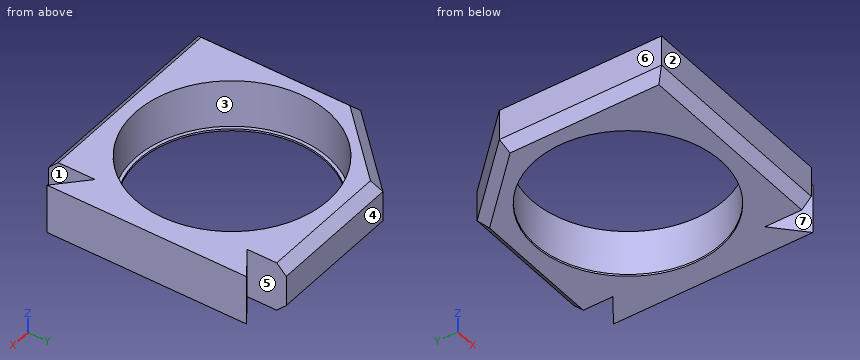
```python
from build123d import *

# Parameters (mm, degrees)
F0_R     = 10.1
F1_DEPTH = 5
F0_R_2   = 9.75
F2_DEPTH = 0.2
F3_SIZE  = 1


with BuildPart() as f1:
    # F0 (on Top) → F1 (new body)
    with BuildSketch(Plane.XY):
        Polygon((-16.0227272727, -12.5188677256), (5.6772727273, -12.5188677256), (5.6772727273, -7.6613227439), (8.6772727273, -10.5188677256), (8.6772727273, 10.3811322744), (5.6772727273, 8.2811322744), (5.6772727273, 12.3811322744), (-8.3227272727, 12.3811322744), (-16.0227272727, 4.4811322744), align=None)
        with Locations((-3.6727272727, -0.0688677256)):
            Circle(F0_R, mode=Mode.SUBTRACT)
    extrude(amount=F1_DEPTH)

    # F0 (on Top) → F2 (join)
    with BuildSketch(Plane.XY):
        Polygon((-16.0227272727, -12.5188677256), (5.6772727273, -12.5188677256), (5.6772727273, -7.6613227439), (8.6772727273, -10.5188677256), (8.6772727273, 10.3811322744), (5.6772727273, 8.2811322744), (5.6772727273, 12.3811322744), (-8.3227272727, 12.3811322744), (-16.0227272727, 4.4811322744), align=None)
        with Locations((-3.6727272727, -0.0688677256)):
            Circle(F0_R, mode=Mode.SUBTRACT)
        with Locations((-3.6727272727, -0.0688677256)):
            Circle(F0_R)
        with Locations((-3.6727272727, -0.0688677256)):
            Circle(F0_R_2, mode=Mode.SUBTRACT)
    extrude(amount=-F2_DEPTH)

    # F3
    f3_edges = [f1.edges().sort_by_distance(p)[0] for p in [
        (-5.172727, -12.518868, 5),
        (-16.022727, -4.018868, 5),
        (-12.172727, 8.431132, 5),
        (-1.322727, 12.381132, 5),
        (-1.322727, 12.381132, -0.2),
        (-12.172727, 8.431132, -0.2),
        (-16.022727, -4.018868, -0.2),
        (-5.172727, -12.518868, -0.2),
    ]]
    chamfer(f3_edges, length=F3_SIZE)


solid = f1.part
```
Check sheet for the modelled part. Datum: model origin and axes. Units: mm. Face numbers are marked on the shaded views. A direction names the side the tool comes from. Give positions to 0.01 mm unless a question says otherwise; leave off trailing zeros. Loops run counter-clockwise (first coordinate to the right, second up) from the corner with the lowest first, then second, coordinate; pieces in that order, holes last. Notation, with made-up numbers: M 86.5,48 L 115.5,48 A21 ccw 115.5,66 Z; hole C 33,6.25 d11. An arc over 180 degrees is marked long. Answer in a Markdown table with one row per item.
1) Cross-section at D-D (y = 5.5). Enter the section's corners in (x, z), plus the area to 3 significant figures.
Solutions:
| item | result |
|---|---|
| outline | M -15.03,0.8 L -13.63,-0.2 L -11.68,-0.2 L -11.68,0 L -12.1,0 L -12.1,5 L -13.63,5 L -15.03,4 Z; M 4.33,-0.2 L 8.68,-0.2 L 8.68,5 L 4.75,5 L 4.75,0 L 4.33,0 Z |
| area | 34.4 mm^2 |
2) Cross-section at C-C (z = 2.9). Enter the section's corners in (x, y), plus the area to 3 significant figures.
Solutions:
| item | result |
|---|---|
| outline | M -16.02,-12.52 L 5.68,-12.52 L 5.68,-7.66 L 8.68,-10.52 L 8.68,10.38 L 5.68,8.28 L 5.68,12.38 L -8.32,12.38 L -16.02,4.48 Z; hole C -3.67,-0.07 d20.2 |
| area | 245 mm^2 |
3) Tool access check on the marked faces 1, 2 and 3. Record the directions out of +Z, -Z, +X, -X, +Y, -Y that give a thin tool (end or side, any length) a straight path to the whole face; none if there is none.
Solutions:
| item | result |
|---|---|
| face 1 | +Z, -Z, -Y |
| face 2 | +Z, -Z, +X, -X, -Y |
| face 3 | +Z |
4) Cross-section at A-A (y = -4.25). Enter the section's corners in (x, z), plus the area to 3 significant figures.
Solutions:
| item | result |
|---|---|
| outline | M -16.02,0.8 L -15.02,-0.2 L -12.48,-0.2 L -12.48,0 L -12.87,0 L -12.87,5 L -15.02,5 L -16.02,4 Z; M 5.14,-0.2 L 8.68,-0.2 L 8.68,5 L 5.52,5 L 5.52,0 L 5.14,0 Z |
| area | 32.0 mm^2 |
5) Mould release check, pull along X, two halves, no side actions. Record for the marked faces 4, 5, 6 and 7: released by +X, released by -X, zero draft, split by the parting line, or undercut.
Solutions:
| item | result |
|---|---|
| face 4 | zero draft |
| face 5 | undercut |
| face 6 | released by -X |
| face 7 | undercut |
6) Cross-section at B-B (x = -3). Enter the section's corners in (y, z).
Solutions:
| item | result |
|---|---|
| outline | M -12.52,0.8 L -11.52,-0.2 L -9.8,-0.2 L -9.8,0 L -10.15,0 L -10.15,5 L -11.52,5 L -12.52,4 Z; M 9.66,-0.2 L 11.38,-0.2 L 12.38,0.8 L 12.38,4 L 11.38,5 L 10.01,5 L 10.01,0 L 9.66,0 Z |
7) Thickness scan on line 1 (Y direction, x = -3.5, z = 2.5); line 2 (X direction, y = -1.5, z = 3.7); line 3 (Z direction, x = 5.75, y = 3.25). Record the ranges inside material, lowest first.
Solutions:
| item | result |
|---|---|
| line 1 | y = -12.52 to -10.17, 10.03 to 12.38 |
| line 2 | x = -16.02 to -13.67, 6.33 to 8.68 |
| line 3 | z = -0.2 to 0 |
